from build123d import *

# Parameters (mm, degrees)
F0_R     = 1.75
F1_DEPTH = 24
F2_R     = 0.5
F3_W     = 8
F3_H     = 7
F4_DEPTH = 15.001


with BuildPart() as f1:
    # F0 (on Top) → F1 (new body)
    with BuildSketch(Plane.XY):
        with BuildLine():
            Line((0, 7), (-13.266499, 7))
            ThreePointArc((-13.266499, 7), (-14.786688, -2.520687), (-10.198039, -11))
            Line((-10.198039, -11), (0, -11))
            Line((0, -11), (0, -15))
            ThreePointArc((0, -15), (15, 0), (0, 15))
            Line((0, 15), (0, 7))
        make_face()
        Circle(F0_R, mode=Mode.SUBTRACT)
    extrude(amount=F1_DEPTH)

    # F2
    f2_edges = [f1.edges().sort_by_distance(p)[0] for p in [
        (0, -15, 12),
    ]]
    fillet(f2_edges, radius=F2_R)

    # F3 (on face) → F4 (cut, through all)
    with BuildSketch(Plane(origin=(0, 0, 0), x_dir=(0, -1, 0), z_dir=(-1, 0, 0))):
        with Locations((-11, 12)):
            Rectangle(F3_W, F3_H)
    extrude(amount=-F4_DEPTH, mode=Mode.SUBTRACT)


solid = f1.part
Work out the finished part from the listing and answer in its coordinate system (mm). A direction names the side the tool comes from. Give positions to 0.01 mm unless a question says otherwise; leave off trailing zeros. Loops run counter-clockwise (first coordinate to the right, second up) from the corner with the lowest first, then second, coordinate; pieces in that order, holes last. Notation, with made-up numbers: (24.25, 48.25) - (40.25, 48.25) arc R19 cw to (40.25, 78.25) - close; hole circle Ø4 at (77, -30.75). An arc over 180 degrees is marked (long way). Answer in a Markdown table with one row per item. Add a question column.
Q1. The part is cut by section B-B (y = 0). Determine the outline of the cut face in (x, z), and give its area (3 significant figures).
Q2. The part is cut by section C-C (z = 12). Determine the outline of the cut face in (x, y), and give its area (3 significant figures).
Q3. Consider line 1 along Z through (x, y) = (2, 11); line 2 along Y through (x, z) = (-8.5, 3.75); line 3 along X through (y, z) = (11.5, 6.5). Determine where each line is inside the solid, lowest interval first.
Q4. Determine the mould class of faces 1 (the flat face through (3, 0, 0)), 2 (the flat face through (-5, -11, 12)), 3 (the cylindrical face through (1.617, -0.67, 11.832)) for opening direction Y: released by +Y, released by -Y, zero draft, split by the parting line, or undercut.
Q5. The part is cut by section D-D (x = 10). Determine the outline of the cut face in (y, z), and give its area (3 significant figures).
Q6. A tool of negligible diameter and unlimited length cuts with its end or side. For faces 4 (the flat face through (0, -13, 12)), 5 (the cylindrical face through (-14.81, -2.39, 11.83)), 6 (the flat face through (5, 10, 8.5)), 7 (the flat face through (3, 0, 24)), 8 (the flat face through (0, 11, 4)), from which of +Z, -Z, +X, -X, +Y, -Y can it reach the whole face along a straight path? Write none if from no direction.
Q7. Each of these flat-tipped pins is pushed along its axis until it touches: P1, Ø4, axis at y = 10, z = 5, coming from the -X side; P2, Ø4, axis at x = 7.5, z = 3.5, coming from the +Y side; P3, Ø12, axis at y = 11, z = 19.5, coming from the +X side; P4, Ø2, axis at x = 0, y = 0, coming from the +Z side. Where does it stop, or does it pass through?
Q8. The part is cut by section A-A (z = 19.25). Determine the outline of the cut face in (x, y).
Solution:
| question | item | result |
|---|---|---|
| 1 | outline | (-15, 0) - (-1.75, 0) - (-1.75, 24) - (-15, 24) - close; (1.75, 0) - (15, 0) - (15, 24) - (1.75, 24) - close |
| 1 | area | 636 mm² |
| 2 | outline | (-13.27, 7) arc R15 ccw to (-10.2, -11) - (0, -11) - (0, -14.49) arc R0.5 ccw to (0.52, -14.99) arc R15 ccw to (13.27, 7) - close; hole circle Ø3.5 at (0, 0) |
| 2 | area | 518 mm² |
| 3 | line 1 | z = 0 to 8.5, 15.5 to 24 |
| 3 | line 2 | y = -11 to 7 |
| 3 | line 3 | x = 0 to 9.63 |
| 4 | face 1 | zero draft |
| 4 | face 2 | released by -Y |
| 4 | face 3 | undercut |
| 5 | outline | (-11.18, 0) - (11.18, 0) - (11.18, 8.5) - (7, 8.5) - (7, 15.5) - (11.18, 15.5) - (11.18, 24) - (-11.18, 24) - close |
| 5 | area | 507 mm² |
| 6 | face 4 | +Z, -Z, -X, -Y |
| 6 | face 5 | +Z, -Z, -X |
| 6 | face 6 | +X, -X, +Y |
| 6 | face 7 | +Z, +X, -X, +Y, -Y |
| 6 | face 8 | +Z, -Z, -X, +Y |
| 7 | P1 | stops at x = 0 |
| 7 | P2 | stops at y = 13.96 |
| 7 | P3 | stops at x = 14.14 |
| 7 | P4 | passes through |
| 8 | outline | (-13.27, 7) arc R15 ccw to (-10.2, -11) - (0, -11) - (0, -14.49) arc R0.5 ccw to (0.52, -14.99) arc R15 ccw to (0, 15) - (0, 7) - close; hole circle Ø3.5 at (0, 0) |
